Input: dimensioned drawing with shaded views. Units: mm. Origin: part minimum x, y, z. A direction names the side the tool comes from. Give positions to 0.01 mm unless a question says otherwise; leave off trailing zeros. Loops run counter-clockwise (first coordinate to the right, second up) from the corner with the lowest first, then second, coordinate; pieces in that order, holes last.
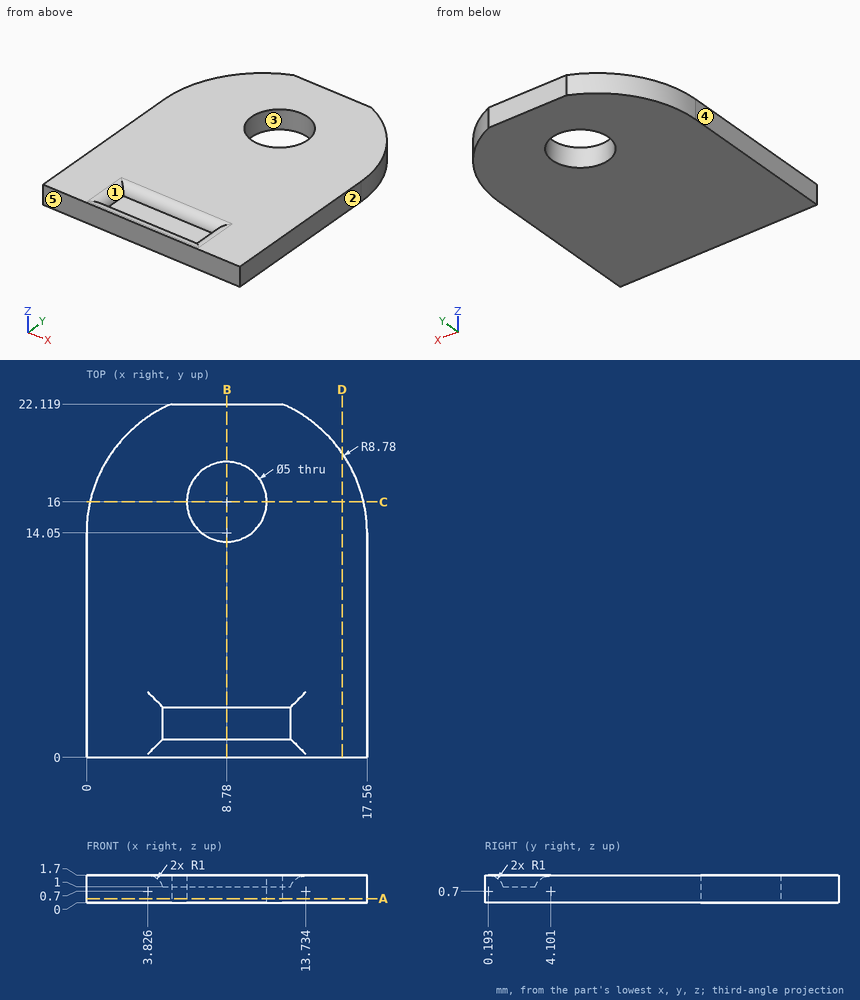
Item 1: Section query C-C on y = 16. Return loops of the section in (x, z), plus the area to 3 significant figures.
Values follow:
outline: (0.22, 0) - (6.28, 0) - (6.28, 1.7) - (0.22, 1.7) - close; (11.28, 0) - (17.34, 0) - (17.34, 1.7) - (11.28, 1.7) - close
area: 20.6 mm2
Item 2: Section query D-D on x = 16. Return loops of the section in (y, z) (1 decimal).
Values follow:
outline: (0, 0) - (19, 0) - (19, 1.7) - (0, 1.7) - close
Item 3: Set-up query: the marked faces 1 and 2. Return all of +Z, -Z, +X, -X, +Y, -Y with unobstructed straight access to the full face (end or side cutting, diameter ignored); none if empty.
Values follow:
face 1: +Z
face 2: +Z, -Z, +X, +Y, -Y
Item 4: Pin query (flat end, axial travel): pin 1 (1.6 mm diameter, centred on x = 8.5, y = 2.5, fed in from +Z). Return the tip coordinate at first contact, or that it passes through.
Values follow:
pin 1: stops at z = 1.3
Item 5: Ray query, probe 1 along Y at (x, z) = (10.25, 1.25) (1 decimal); probe 2 along Y at (x, z) = (7.25, 1.45) (1 decimal); probe 3 along Y at (x, z) = (9, 0.35). Return the intervals inside material, ascending.
Values follow:
probe 1: y = 0 to 1, 3.3 to 14, 18 to 22.1
probe 2: y = 0 to 0.9, 3.4 to 14, 18 to 22.1
probe 3: y = 0 to 13.51, 18.49 to 22.12
Item 6: Section query A-A on z = 0.25. Return loops of the section in (x, y).
Values follow:
outline: (0, 0) - (17.56, 0) - (17.56, 14.05) arc R8.78 ccw to (12.24, 22.12) - (5.32, 22.12) arc R8.78 ccw to (0, 14.05) - close; hole circle Ø5 at (8.78, 16)
Item 7: Section query B-B on x = 8.78. Return loops of the section in (y, z).
Values follow:
outline: (0, 0) - (13.5, 0) - (13.5, 1.7) - (4.1, 1.7) arc R1 ccw to (3.15, 1) - (1.15, 1) arc R1 ccw to (0.19, 1.7) - (0, 1.7) - close; (18.5, 0) - (22.12, 0) - (22.12, 1.7) - (18.5, 1.7) - close
Item 8: Draft query along Y for the marked faces 3, 4 and 5. Return one class per face: +Y half, -Y half, draft (parallel to the pull), parting line (faces both ways), or undercut.
Values follow:
face 3: undercut
face 4: draft
face 5: -Y half
